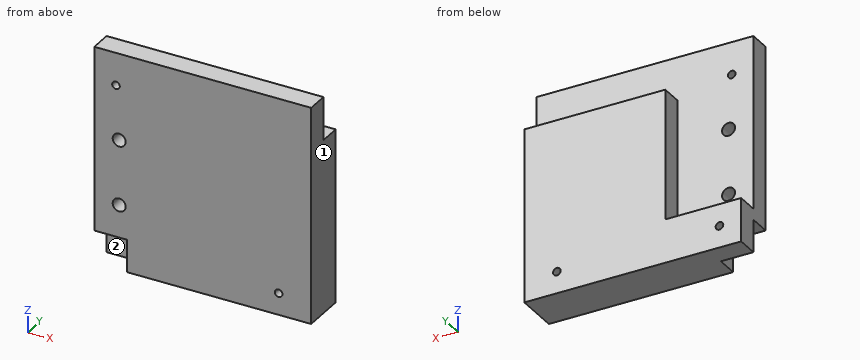
Autodesk Inventor part; units mm, degrees
ref_plane "YZ Plane" through (0, 0, 0) normal (1, 0, 0) x (0, 1, 0)
ref_plane "XZ Plane" through (0, 0, 0) normal (0, 1, 0) x (-1, 0, 0)
ref_plane "XY Plane" through (0, 0, 0) normal (0, 0, 1) x (1, 0, 0)
sketch "Boceto1" plane through (0, 0, 0) normal (0, 1, 0) x (-1, 0, 0)
  line L0 (100, 100) -> (-100, 100)
  line L1 (-100, 100) -> (-100, -100)
  line L2 (-100, -100) -> (100, -100)
  line L3 (100, -100) -> (100, 100)
  line L4 (100, 100) -> (-100, -100) construction
  line L5 (-100, 100) -> (100, -100) construction
  point P0 (0, 0)
  dimension "d0" = 200
  dimension "d1" = 200
extrude "Extrusión1" add sketch "Boceto1" along normal blind 20
sketch "Boceto2" plane through (0, 20, 0) normal (0, 1, 0) x (1, 0, 0)
  circle A0 centre (-11.5239, -30.0616) radius 3
  circle A1 centre (11.4761, -30.0616) radius 3
  circle A2 centre (-11.5239, -60.0616) radius 3
  circle A3 centre (11.4761, -60.0616) radius 3
  line L0 (-0.0239, -45.0616) -> (-35.0239, -45.0616)
  line L1 (-35.0239, -45.0616) -> (-35.0239, -80.0616)
  line L2 (-0.0239, -45.0616) -> (34.9761, -45.0616)
  line L3 (-11.5239, -30.0616) -> (11.4761, -60.0616)
  line L4 (-11.5239, -60.0616) -> (11.4761, -30.0616)
  line L5 (34.9761, -20.0616) -> (-35.0239, -20.0616)
  line L6 (-35.0239, -20.0616) -> (-35.0239, -80.0616)
  line L7 (34.9761, -80.0616) -> (34.9761, -20.0616)
  line L8 (-105, -100.0616) -> (105, -100.0616)
  line L9 (-105.0239, -80.0616) -> (104.9761, -80.0616)
  line L10 (-35.0239, -80.0616) -> (34.9761, -80.0616)
  line L11 (105, -100.0616) -> (95.8154, -100.0616)
  line L12 (-105.0239, -80.0616) -> (104.9761, -80.0616)
  line L13 (105, -80.0616) -> (-105, -80.0616)
  line L14 (-105, -100.0616) -> (105, -100.0616)
  line L15 (105, -90.0616) -> (94.0798, -90.0616)
  line L16 (-105, -100.0616) -> (105, -100.0616)
  line L17 (-105, -80.0616) -> (105, -80.0616)
  line L18 (105, -80.0616) -> (105, -100.0616)
  line L19 (105, -100.0616) -> (-105, -100.0616)
  line L20 (-105, -100.0616) -> (-105, -80.0616)
  line L21 (-100, 100) -> (-100, -100)
  line L22 (-100, -100) -> (100.4077, -100)
  point P0 (0, 0)
  point P1 (0, -10.0616)
  point P2 (0, -90.0616)
  point P3 (-0.0478, -80.0616)
  dimension "d4" = 20
  dimension "d5" = 20
  dimension "d6" = 30
  dimension "d7" = 30
  dimension "d8" = 20
  dimension "d9" = 35
  dimension "d10" = 35
  dimension "d11" = 60
extrude "Extrusión2" cut sketch "Boceto2" against normal blind 10
sketch "Boceto3" plane through (0, 20, 0) normal (0, 1, 0) x (1, 0, 0)
  circle A0 centre (-11.5239, -30.0616) radius 3
  circle A1 centre (-11.5239, -30.0616) radius 3
  circle A2 centre (11.4761, -30.0616) radius 3
  circle A3 centre (11.4761, -30.0616) radius 3
  circle A4 centre (11.4761, -60.0616) radius 3
  circle A5 centre (11.4761, -60.0616) radius 3
  circle A6 centre (-11.5239, -60.0616) radius 3
  point P0 (0, 0)
extrude "Extrusión3" cut sketch "Boceto3" against normal blind 20
sketch "Boceto4" plane through (0, 20, 0) normal (0, 1, 0) x (1, 0, 0)
  circle A0 centre (-51.75, 78.25) radius 1.75
  line L0 (-50, 70) -> (-60, 70)
  line L1 (-60, 70) -> (-60, 80)
  line L2 (-60, 80) -> (-50, 80)
  line L3 (-50, 80) -> (-50, 70)
  line L4 (-50, 70) -> (-60, 80) construction
  line L5 (-60, 70) -> (-50, 80) construction
  line L6 (-105, 90) -> (-105, -90)
  circle A1 centre (-58.25, 71.75) radius 1.75
  line L7 (0, 90) -> (0, 77.3124)
  circle A2 centre (51.75, 78.25) radius 1.75
  line L8 (50, 70) -> (60, 70)
  line L9 (60, 70) -> (60, 80)
  line L10 (60, 80) -> (50, 80)
  line L11 (50, 80) -> (50, 70)
  line L12 (50, 70) -> (60, 80) construction
  line L13 (60, 70) -> (50, 80) construction
  circle A3 centre (58.25, 71.75) radius 1.75
  line L14 (100, 100) -> (-100, 100)
  line L15 (-100, 100) -> (-100, -80.0616)
  line L16 (100, -80.0616) -> (100, 100)
  point P0 (0, 0)
  point P1 (0, 0)
  point P2 (-60, 75)
  point P3 (60, 75)
  dimension "d16" = 3.5
  dimension "d18" = 1.75
  dimension "d19" = 1.75
  dimension "d20" = 1.75
  dimension "d21" = 1.75
  dimension "d22" = 10
  dimension "d23" = 10
  dimension "d25" = 20
  dimension "d26" = 40
  dimension "d27" = 40
hole "Agujero1" at (-58.25, 20, -71.75) at (-51.75, 20, -78.25) at (58.25, 20, -71.75) at (51.75, 20, -78.25) direction (0, -1, 0) diameter 3.5 end through all
sketch "Boceto5" plane through (0, 20, 0) normal (0, 1, 0) x (1, 0, 0)
  line L0 (0, 90) -> (0, 68.25)
  circle A0 centre (-51.75, 78.25) radius 1.75
  line L1 (-50, 78.25) -> (-50, 100)
  circle A1 centre (-58.25, 71.75) radius 1.75
  line L2 (-60, 71.75) -> (-60, 100)
  line L3 (-60, 100) -> (-70, 100)
  line L4 (-50, 100) -> (-40, 100)
  line L5 (-40, 100) -> (-40, 60)
  line L6 (-40, 60) -> (-70, 60)
  line L7 (-70, 60) -> (-70, 100)
  line L8 (-70, 100) -> (-40, 100)
  circle A2 centre (51.75, 78.25) radius 1.75
  line L9 (50, 78.25) -> (50, 100)
  circle A3 centre (58.25, 71.75) radius 1.75
  line L10 (60, 71.75) -> (60, 100)
  line L11 (60, 100) -> (70, 100)
  line L12 (50, 100) -> (40, 100)
  line L13 (40, 100) -> (40, 60)
  line L14 (40, 60) -> (70, 60)
  line L15 (70, 60) -> (70, 100)
  line L16 (70, 100) -> (40, 100)
  point P0 (0, 0)
  dimension "d38" = 10
  dimension "d39" = 10
  dimension "d40" = 40
extrude "Extrusión4" cut sketch "Boceto5" against normal blind 10
ref_plane "Plano de trabajo1" through (0, 0, -100) normal (-1, 0, 0) x (0, 0, 1)
ref_plane "Plano de trabajo2" through (100, 0, 0) normal (0, 0, -1) x (-1, 0, 0)
sketch "Boceto7" plane through (0, 0, 0) normal (0, -1, 0) x (1, 0, 0)
  circle A0 centre (10, -10) radius 1.75
  line L0 (6.803, 0) -> (14.6069, 0)
  line L1 (0, 0) -> (0, -4.8284)
  line L2 (0, 0) -> (20.0354, 0)
  circle A1 centre (10, 10) radius 1.75
  line L3 (0, 0) -> (0, 4.8284)
  circle A2 centre (-10, -10) radius 1.75
  circle A3 centre (-10, 10) radius 1.75
  dimension "d52" = 3.5
  dimension "d54" = 10
  dimension "d55" = 10
hole "Agujero2" at (10, 0, -10) at (10, 0, 10) at (-10, 0, 10) at (-10, 0, -10) direction (0, 1, 0) diameter 3.5 end through all
sketch "Boceto8" plane through (0, 0, 0) normal (0, -1, 0) x (1, 0, 0)
  line L0 (-15, 15) -> (15, 15)
  line L1 (15, 15) -> (15, -15)
  line L2 (15, -15) -> (-15, -15)
  line L3 (-15, -15) -> (-15, 15)
  line L4 (-15, 15) -> (15, -15) construction
  line L5 (15, 15) -> (-15, -15) construction
  point P0 (0, 0)
  dimension "d63" = 30
  dimension "d64" = 30
extrude "Extrusión5" cut sketch "Boceto8" against normal blind 10
sketch "Boceto9" plane through (0, 0, 0) normal (0, -1, 0) x (1, 0, 0)
  circle A0 centre (85, -10) radius 1.75
  line L0 (100, 100) -> (100, -100)
  line L1 (140, 0) -> (-140, 0)
  circle A1 centre (85, 10) radius 1.75
  line L2 (0, 0) -> (0, 9.4908)
  circle A2 centre (-85, -10) radius 1.75
  circle A3 centre (-85, 10) radius 1.75
  line L3 (0, 0) -> (6.3157, 6.3157)
  line L4 (0, 0) -> (8.9318, 0) construction
  circle A4 centre (10, 85) radius 1.75
  circle A5 centre (-10, -85) radius 1.75
  line L5 (0, 0) -> (5.9531, -5.9531)
  line L6 (0, 0) -> (8.419, 0) construction
  circle A6 centre (10, -85) radius 1.75
  circle A7 centre (-10, 85) radius 1.75
  dimension "d67" = 3.5
  dimension "d68" = 15
  dimension "d69" = 10
  dimension "d70" = 45
  dimension "d71" = 45
hole "Agujero3" at (-10, 0, 85) at (10, 0, 85) at (85, 0, 10) at (85, 0, -10) at (-85, 0, 10) at (-85, 0, -10) at (-10, 0, -85) at (10, 0, -85) direction (0, 1, 0) diameter 3.5 end through all
split "Dividir3" plane through (100, 0, 0) removes the side toward (0, 0, -1)
split "Dividir4" plane through (0, 0, -100) removes the side toward (-1, 0, 0)
properties part number "base_front_4"
Geometry: final body of the model. Coordinates: model frame, mm. Face numbers are marked on the shaded views. A direction names the side the tool comes from. Give positions to 0.01 mm unless a question says otherwise; leave off trailing zeros. Write each loop counter-clockwise with the first axis right and the second up, starting at its lowest first coordinate (ties: lowest second). Pieces come first, ordered by that corner, then holes.
(1) Cut plane C-C, the plane z = 85. Return loops of the section in (x, y).
(2) Ray query, line 1 (X direction, y = 13, z = 10); line 2 (Z direction, x = 85, y = 14.5); line 3 (X direction, y = 9, z = 85). Return the intervals inside material, ascending.
(3) First-contact query: P1, Ø5, axis at x = 11.48, z = 60.06, coming from the +Y side; P2, Ø3, axis at x = 7, y = 4, coming from the -Z side; P3, Ø9.5, axis at x = 11.48, z = 30.06, coming from the +Y side; P4, Ø5, axis at x = 24.5, y = 17.5, coming from the +Z side. Flat tips, straight axial feed; report the tip coordinate or a pass-through.
(4) Cut plane D-D, the plane x = 85. Return loops of the section in (y, z), then the cut area to 3 significant figures.
(5) Access query for the marked faces 1 and 2. Directions: +Z, -Z, +X, -X, +Y, -Y. A direction counts if a zero-diameter tool reaches every point of the face in a straight line with its end or side. Return the directions, or none.
(6) Cut plane B-B, the plane y = 11.75. Return loops of the section in (x, z).
(7) Cut plane A-A, the plane z = 10. Return loops of the section in (x, y), then the cut area to 4 significant figures.
Values follow:
1. outline: (0, 0) - (8.25, 0) - (8.25, 10) - (0, 10) - close; (11.75, 0) - (100, 0) - (100, 10) - (11.75, 10) - close
2. line 1: x = 0 to 8.25, 11.75 to 83.25, 86.75 to 100
2. line 2: z = 0 to 8.25, 11.75 to 80.06
2. line 3: x = 0 to 8.25, 11.75 to 100
3. P1: passes through
3. P2: stops at z = 15
3. P3: stops at y = 10
3. P4: stops at z = 20.06
4. outline: (0, 0) - (20, 0) - (20, 8.25) - (0, 8.25) - close; (0, 11.75) - (20, 11.75) - (20, 80.06) - (10, 80.06) - (10, 100) - (0, 100) - close
4. area: 1,730 mm2
5. face 1: +Z, -Z, +X, +Y, -Y
5. face 2: -Z, -X, -Y
6. outline: (0, 0) - (100, 0) - (100, 80.06) - (34.98, 80.06) - (34.98, 20.06) - (0, 20.06) - close; hole circle Ø3.5 at (10, 10); hole circle Ø3.5 at (85, 10)
7. outline: (0, 10) - (8.25, 10) - (8.25, 20) - (0, 20) - close; (11.75, 10) - (15, 10) - (15, 0) - (83.25, 0) - (83.25, 20) - (11.75, 20) - close; (86.75, 0) - (100, 0) - (100, 20) - (86.75, 20) - close
7. area: 1,745 mm2
